Source: CAD feature listing. Evaluate the final solid. Frame: model axes, mm. A direction names the side the tool comes from. Give positions to 0.01 mm unless a question says otherwise; leave off trailing zeros. Order: outer loops, then holes, each group sorted by start corner. A loop starts at its lowest first (then second) coordinate and runs counter-clockwise, first axis right, second up. Notation, with made-up numbers: (65.5, 8) - (107.5, 8) arc R12 ccw to (107.5, 23) - close; hole circle Ø11 at (22.5, 27.25). An arc over 180 degrees is marked (long way). Write each question's results on one line, items separated by ' | '. Start each with the question number.
Item 1: Line query: line 1 along Y through (x, z) = (3, 10.75); line 2 along Z through (x, y) = (0, -23.55); line 3 along Y through (x, z) = (0, 12.5). Output: solid intervals per line, ascending.
Item 2: Section B-B on y = -14. Output: boundary loops of the cut face in (x, z), and give its area (3 significant figures).
Item 3: Section A-A on x = 0. Output: boundary loops of the cut face in (y, z).
Item 4: Section D-D on z = 9.5. Output: boundary loops of the cut face in (x, y).
Item 5: Set-up query: faces 4 (the cylindrical face through (5.5, -23.49, 8.43)), 5 (the flat face through (-2.5, 41, 13)), 6 (the flat face through (9, -23, 13)). Return all of +Z, -Z, +X, -X, +Y, -Y with unobstructed straight access to the full face (end or side cutting, diameter ignored); none if empty.
Item 6: Mould query, pull axis Y, two halves, no side actions, for faces 1 (the flat face through (-9, -23, 13)), 2 (the flat face through (-5, -6, 12)), 3 (the flat face through (-7, 40, 13)). Classes: released by +Y, released by -Y, zero draft, split by the parting line, or undercut.
Item 7: Contact query for flat-ended pins moving along their axis: pin 1 Ø0.5 at (y, z) = (-23.5, 13) entering from +X; pin 2 Ø1.1 at (x, y) = (-0.5, -23.5) entering from -Z; pin 3 Ø5 at (x, y) = (-3.5, 20) entering from -Z. Output: stop coordinate, or through.
Item 8: Section C-C on y = 7. Output: boundary loops of the cut face in (x, z), and give its area (3 significant figures).
```python
from build123d import *

# Parameters (mm, degrees)
BOSS_EXTRUDE1_DEPTH = 32
SKETCH2_W           = 13.568258361
SKETCH2_H           = 32
CUT_EXTRUDE1_DEPTH  = 2.1
SKETCH3_W           = 23.8
SKETCH3_H           = 2
BOSS_EXTRUDE2_DEPTH = 23
SKETCH4_W           = 23.8
SKETCH4_H           = 2
BOSS_EXTRUDE3_DEPTH = 8
CUT_EXTRUDE2_REACH  = 15.568
SKETCH5_R           = 7
SKETCH6_W           = 2.5
SKETCH6_H           = 2
BOSS_EXTRUDE4_DEPTH = 2
SKETCH7_W           = 7
SKETCH7_H           = 2
BOSS_EXTRUDE5_DEPTH = 1
BOSS_EXTRUDE6_START = -2
SKETCH8_W           = 14
SKETCH8_H           = 1
BOSS_EXTRUDE6_DEPTH = 5
CUT_EXTRUDE3_REACH  = 68
SKETCH9_R           = 1.5
FILLET1_R           = 5


with BuildPart() as part:
    # Sketch1 → Boss-Extrude1 (new body)
    with BuildSketch(Plane(origin=(0, 0, 0), x_dir=(1, 0, 0), z_dir=(0, 1, 0))):
        with BuildLine():
            Line((14, -0.431741639), (11.721082209, -0.431741639))
            ThreePointArc((11.721082209, -0.431741639), (10.883203702, -4.783711919), (8.489359235, -8.513483277))
            Line((8.489359235, -8.513483277), (-8.489359235, -8.513483277))
            ThreePointArc((-8.489359235, -8.513483277), (-10.883203702, -4.783711919), (-11.721082209, -0.431741639))
            Line((-11.721082209, -0.431741639), (-14, -0.431741639))
            Line((-14, -0.431741639), (-14, -14))
            Line((-14, -14), (14, -14))
            Line((14, -14), (14, -0.431741639))
        make_face()
    extrude(amount=BOSS_EXTRUDE1_DEPTH)

    # Sketch2 → Cut-Extrude1 (cut)
    with BuildSketch(Plane.ZY.offset(14)):
        with Locations((7.21587082, 16)):
            Rectangle(SKETCH2_W, SKETCH2_H)
    cut_extrude1 = extrude(amount=-CUT_EXTRUDE1_DEPTH, mode=Mode.SUBTRACT)

    # Mirror1: Cut-Extrude1 across plane
    add(cut_extrude1.mirror(Plane(origin=(0, 0, 0), x_dir=(0, 0, 1), z_dir=(1, 0, 0))), mode=Mode.SUBTRACT)

    # Sketch3 → Boss-Extrude2 (add)
    with BuildSketch(Plane.XZ):
        with Locations((0, 13)):
            Rectangle(SKETCH3_W, SKETCH3_H)
    extrude(amount=BOSS_EXTRUDE2_DEPTH)

    # Sketch4 → Boss-Extrude3 (add)
    with BuildSketch(Plane(origin=(0, 32, 0), x_dir=(1, 0, 0), z_dir=(0, 1, 0))):
        with Locations((0, -13)):
            Rectangle(SKETCH4_W, SKETCH4_H)
    extrude(amount=BOSS_EXTRUDE3_DEPTH)

    # Sketch5 → Cut-Extrude2 (cut, up to next)
    with BuildSketch(Plane.XY.offset(14), mode=Mode.PRIVATE) as cut_extrude2_sk1:
        with Locations((0, -11.97008474)):
            Circle(SKETCH5_R)
    cut_extrude2_tool1 = extrude(cut_extrude2_sk1.sketch, amount=-CUT_EXTRUDE2_REACH, mode=Mode.PRIVATE) & part.part
    add(cut_extrude2_tool1.solids().sort_by_distance((0, -11.970085, 14))[0], mode=Mode.SUBTRACT)

    # Sketch6 → Boss-Extrude4 (add)
    with BuildSketch(Plane(origin=(0, 40, 0), x_dir=(1, 0, 0), z_dir=(0, 1, 0))):
        with Locations((-1.25, -13)):
            Rectangle(SKETCH6_W, SKETCH6_H)
        with Locations((1.25, -13)):
            Rectangle(SKETCH6_W, SKETCH6_H)
    extrude(amount=BOSS_EXTRUDE4_DEPTH)

    # Sketch7 → Boss-Extrude5 (add)
    with BuildSketch(Plane.XZ.offset(23)):
        with Locations((3.5, 13)):
            Rectangle(SKETCH7_W, SKETCH7_H)
        with Locations((-3.5, 13)):
            Rectangle(SKETCH7_W, SKETCH7_H)
    extrude(amount=BOSS_EXTRUDE5_DEPTH)

    # Sketch8 → Boss-Extrude6 (add)
    with BuildSketch(Plane.XY.offset(14).offset(BOSS_EXTRUDE6_START)):
        with Locations((0, -23.5)):
            Rectangle(SKETCH8_W, SKETCH8_H)
    extrude(amount=-BOSS_EXTRUDE6_DEPTH)

    # Sketch9 → Cut-Extrude3 (cut, up to next)
    with BuildSketch(Plane.XZ.offset(24), mode=Mode.PRIVATE) as cut_extrude3_sk1:
        with Locations((0, 9.5)):
            Circle(SKETCH9_R)
    cut_extrude3_tool1 = extrude(cut_extrude3_sk1.sketch, amount=-CUT_EXTRUDE3_REACH, mode=Mode.PRIVATE) & part.part
    add(cut_extrude3_tool1.solids().sort_by_distance((0, -24, 9.5))[0], mode=Mode.SUBTRACT)

    # Fillet1
    fillet1_edges = [part.edges().sort_by_distance(p)[0] for p in [
        (-7, -23.5, 7),
        (7, -23.5, 7),
    ]]
    fillet(fillet1_edges, radius=FILLET1_R)


solid = part.part
```
Evaluation:
1) line 1: y = -24 to -23, 0 to 32 | line 2: z = 7 to 8, 11 to 14 | line 3: y = -24 to -18.97, -4.97 to 42
2) outline: (-11.9, 12) - (-6.7, 12) - (-6.7, 14) - (-11.9, 14) - close; (6.7, 12) - (11.9, 12) - (11.9, 14) - (6.7, 14) - close | area: 20.8 mm^2
3) outline: (-24, 7) - (-23, 7) - (-23, 8) - (-24, 8) - close; (-24, 11) - (-23, 11) - (-23, 12) - (-18.97, 12) - (-18.97, 14) - (-24, 14) - close; (-4.97, 12) - (0, 12) - (0, 8.51) - (32, 8.51) - (32, 12) - (42, 12) - (42, 14) - (-4.97, 14) - close
4) outline: (-11.9, 0) - (11.9, 0) - (11.9, 32) - (-11.9, 32) - close; (-6.33, -24) - (-1.5, -24) - (-1.5, -23) - (-6.33, -23) - close; (1.5, -24) - (6.33, -24) - (6.33, -23) - (1.5, -23) - close
5) face 4: -Z, +X, -Y | face 5: +Z, -Z, -X, +Y | face 6: +Z, -Z, +X, -Y
6) face 1: released by -Y | face 2: undercut | face 3: released by +Y
7) pin 1: stops at x = 7 | pin 2: stops at z = 7 | pin 3: stops at z = 8.51
8) outline: (-11.9, 0.43) - (-11.72, 0.43) arc R11.72 cw to (-8.49, 8.51) - (8.49, 8.51) arc R11.72 cw to (11.72, 0.43) - (11.9, 0.43) - (11.9, 14) - (-11.9, 14) - close | area: 150 mm^2
